Autodesk Inventor part; units mm, degrees
ref_plane "YZ Plane" through (0, 0, 0) normal (1, 0, 0) x (0, 1, 0)
ref_plane "XZ Plane" through (0, 0, 0) normal (0, 1, 0) x (-1, 0, 0)
ref_plane "XY Plane" through (0, 0, 0) normal (0, 0, 1) x (1, 0, 0)
sketch "Sketch1" plane through (0, 0, 0) normal (0, 0, 1) x (1, 0, 0)
  line L0 (-40, -40) -> (-40, 40) construction
  line L1 (40, -40) -> (-40, -40) construction
  line L2 (40, 40) -> (40, -40) construction
  circle A0 centre (35.75, -35.75) radius 2.25 construction
  circle A1 centre (-35.75, -35.75) radius 2.25 construction
  circle A2 centre (0, 0) radius 35.75 construction
  line L3 (-40, -40) -> (-25, -55)
  line L4 (-40, -40) -> (-18.7868, -40) construction
  line L5 (-25, -55) -> (25, -55)
  line L6 (25, -55) -> (40, -40)
  line L7 (-40, -40) -> (-40, -30.4857)
  line L8 (40, -40) -> (40, -30.4857)
  circle A3 centre (0, 0) radius 38.75 construction
  circle A4 centre (35.75, -35.75) radius 2.25
  circle A5 centre (-35.75, -35.75) radius 2.25
  line L9 (-40, -30.4857) -> (-18.673, -30.4857)
  line L10 (40, -30.4857) -> (18.673, -30.4857)
  arc A6 (-18.673, -30.4857) -> (18.673, -30.4857) centre (0, 0) ccw
extrude "Extrusion3" add sketch "Sketch1" along normal blind 2.5
sketch "Sketch5" plane through (-25, -55, 0) normal (0, -1, 0) x (1, 0, 0)
  line L0 (50, 2.5) -> (0, 2.5)
  line L1 (0, 2.5) -> (0, -26.5)
  line L2 (0, -26.5) -> (50, -26.5)
  line L3 (50, -26.5) -> (50, 2.5)
  point P0 (25, 0)
  dimension "d22" = 29
extrude "Extrusion5" add sketch "Sketch5" along normal blind 2.5
sketch "Sketch6" plane through (-25, -55, 0) normal (0, 1, 0) x (1, 0, 0)
  line L0 (40, 14) -> (10, 14)
  point P0 (25, 0)
  point P1 (25, 0)
  point P2 (25, 14)
  dimension "d25" = 30
  dimension "d52" = 14
hole "Hole2" at (15, -55, -14) at (-15, -55, -14) direction (0, -1, 0) diameter 4.5 end through all
fillet "Fillet2" radius 2 2 edges at (40, -30.4857, 1.25) (-40, -30.4857, 1.25)
sketch "Sketch8" plane through (0, 0, 0) normal (0, 0, -1) x (-1, 0, 0)
  line L0 (-40, -40) -> (40, -40) construction
  line L1 (-40, 40) -> (-40, -40) construction
  line L2 (40, 40) -> (-40, 40) construction
  line L3 (40, -40) -> (40, 40) construction
  circle A0 centre (35.75, -35.75) radius 2.25 construction
  circle A1 centre (35.75, 35.75) radius 2.25 construction
  circle A2 centre (-35.75, 35.75) radius 2.25 construction
  circle A3 centre (-35.75, -35.75) radius 2.25 construction
  circle A4 centre (0, 0) radius 38.75 construction
  line L4 (-25, -55) -> (-22.5, -55)
  line L5 (-22.5, -55) -> (-22.5, -40)
  line L6 (-22.5, -40) -> (-25, -40)
  line L7 (-25, -40) -> (-25, -55)
  line L8 (25, -55) -> (22.5, -55)
  line L9 (22.5, -55) -> (22.5, -40)
  line L10 (22.5, -40) -> (25, -40)
  line L11 (25, -40) -> (25, -55)
  line L12 (25, -55) -> (-25, -55)
  line L13 (1.25, -55) -> (-1.25, -55)
  line L14 (-1.25, -55) -> (-1.25, -40)
  line L15 (-1.25, -40) -> (1.25, -40)
  line L16 (1.25, -40) -> (1.25, -55)
  point P0 (0, -40)
  dimension "d39" = 2.5
  dimension "d40" = 2.5
  dimension "d41" = 2.5
extrude "Extrusion7" add sketch "Sketch8" along normal up to surface (26.5 mm away)
sketch "Sketch9" plane through (-25, -57.5, 0) normal (0, -1, 0) x (1, 0, 0)
  line L0 (23.75, 0) -> (23.75, -26.5) construction
  line L1 (23.75, 0) -> (23.75, -26.5) construction
  circle A0 centre (40, -14) radius 2.25 construction
  circle A1 centre (10, -14) radius 2.25 construction
  line L2 (40, -14) -> (10, -14) construction
  line L3 (23.75, -26.5) -> (21.75, -26.5)
  line L4 (21.75, -26.5) -> (21.75, -14)
  line L5 (21.75, -14) -> (23.75, -14)
  line L6 (23.75, -14) -> (23.75, -26.5)
  point P0 (25, 0)
  dimension "d45" = 2
extrude "Extrusion8" cut sketch "Sketch9" against normal through all
fillet "Fillet3" radius 1 2 edges at (-1.25, -56.25, -14) (-3.25, -56.25, -14)
fillet "Fillet4" radius 2 1 edges at (-3.25, -56.25, -26.5)
equation "\"d23\" = ep"
equation "\"d39\" = ep"
equation "\"d40\" = ep"
equation "\"d41\" = ep"
equation "\"d42\" = ep"
equation "\"d46\" = ep"
equation "\"d44\" = A1"
properties part number "support"
Geometry: final body of the model. Coordinates: model frame, mm. A direction names the side the tool comes from. Round coordinates to 2 decimals unless told otherwise and drop trailing zeros. Write each loop counter-clockwise with the first axis right and the second up, starting at its lowest first coordinate (ties: lowest second). Pieces come first, ordered by that corner, then holes. Notation, with made-up numbers: M -24.75,56 L -16.75,56 A15 cw -16.75,61 Z; hole C 54.5,86 d4. An arc over 180 degrees is marked long. Answer in a Markdown table with one row per item. Add a question column.
(1) Contact query for flat-ended pins moving along their axis: pin 1 (1 mm diameter, centred on x = -16.5, y = -44, fed in from -Z); pin 2 (1 mm diameter, centred on x = 26.5, z = -19, fed in from -Y); pin 3 (1.5 mm diameter, centred on x = 18, z = -8.5, fed in from +Y); pin 4 (12 mm diameter, centred on y = -50, z = -9, fed in from +X). Output: stop coordinate, or through.
(2) Draft query along Z for faces 5 (the face through (16.996, -56.268, -12.962)), 6 (the face through (-1, -44, 2.5)), 7 (the face through (-18.7, -55.2, -26.5)), 8 (the face through (1.25, -48, -13)). Return one class per face: pulls with the +Z half, pulls with the -Z half, needs draft (parallel to the pull), parting line crosses it, or undercut.
(3) Cut plane D-D, the plane y = -36.5. Return the cut outline in (x, z), then the cut area to 3 significant figures.
(4) Cut plane B-B, the plane x = -15. Return the cut outline in (y, z), then the cut area to 3 significant figures.
(5) Ray query, L1, parallel to X at y = -45.25, z = -11; L2, parallel to Z at x = -13.5, y = -43.5; L3, parallel to Y at x = 18.5, z = -25.25. Return the intervals inside material, ascending.
(6) Cut plane C-C, the plane y = -46.5. Return the cut outline in (x, z).
(7) Reachability of faces 1 (the face through (-3.82, -56.23, -25.9)), 2 (the face through (-12, -55, -13)), 3 (the face through (-39.4, -31.06, 1.27)), 4 (the face through (-24, -40, -13)) from +Z, -Z, +X, -X, +Y, -Y: full face, straight path, thin tool, end or side. Return the list, or none.
(8) Cut plane A-A, the plane z = -19.75. Return the cut outline in (x, y).
Established:
| question | item | result |
|---|---|---|
| 1 | pin 1 | z = 0 |
| 1 | pin 2 | through |
| 1 | pin 3 | y = -55 |
| 1 | pin 4 | x = 25 |
| 2 | face 5 | undercut |
| 2 | face 6 | pulls with the +Z half |
| 2 | face 7 | pulls with the -Z half |
| 2 | face 8 | needs draft |
| 3 | outline | M -40,0 L -37.87,0 L -37.87,2.5 L -40,2.5 Z; M -33.63,0 L 33.63,0 L 33.63,2.5 L -33.63,2.5 Z; M 37.87,0 L 40,0 L 40,2.5 L 37.87,2.5 Z |
| 3 | area | 179 mm² |
| 4 | outline | M -57.5,-26.5 L -55,-26.5 L -55,-16.25 L -57.5,-16.25 Z; M -57.5,-11.75 L -55,-11.75 L -55,0 L -32.45,0 L -32.45,2.5 L -57.5,2.5 Z |
| 4 | area | 118 mm² |
| 5 | L1 | -25 to -22.5, -1.25 to 1.25, 22.5 to 25 |
| 5 | L2 | 0 to 2.5 |
| 5 | L3 | -57.5 to -55 |
| 6 | outline | M -33.5,0 L -25,0 L -25,-26.5 L -22.5,-26.5 L -22.5,0 L -1.25,0 L -1.25,-26.5 L 1.25,-26.5 L 1.25,0 L 22.5,0 L 22.5,-26.5 L 25,-26.5 L 25,0 L 33.5,0 L 33.5,2.5 L -33.5,2.5 Z |
| 7 | face 1 | -Z, +Y, -Y |
| 7 | face 2 | -Z, +Y |
| 7 | face 3 | +Z, -Z, -X, +Y |
| 7 | face 4 | -Z, +X, -X, +Y |
| 8 | outline | M -25,-57.5 L -3.25,-57.5 L -3.25,-55 L -22.5,-55 L -22.5,-40 L -25,-40 Z; M -1.25,-57.5 L 25,-57.5 L 25,-40 L 22.5,-40 L 22.5,-55 L 1.25,-55 L 1.25,-40 L -1.25,-40 Z |
